from build123d import *

# Parameters (mm, degrees)
SKETCH1_R           = 11
SKETCH1_R_2         = 10
SKETCH1_R_3         = 1.75
SKETCH1_W           = 4
SKETCH1_H           = 20
BOSS_EXTRUDE1_DEPTH = 4


with BuildPart() as part:
    # Sketch1 → Boss-Extrude1 (new body)
    with BuildSketch(Plane(origin=(0, 0, 0), x_dir=(0, 0, -1), z_dir=(1, 0, 0))):
        Polygon((-20, 170.087118875), (20, 170.087118875), (75, 72.036415883), (75, -3.912881125), (55, -3.912881125), (55, 0.087118875), (10, 0.087118875), (10, -3.912881125), (-10, -3.912881125), (-10, 0.087118875), (-55, 0.087118875), (-55, -3.912881125), (-75, -3.912881125), (-75, 72.036415883), align=None)
        with Locations((0, 30.087118875)):
            Circle(SKETCH1_R, mode=Mode.SUBTRACT)
        with Locations((0, 140.087118875)):
            Circle(SKETCH1_R_2, mode=Mode.SUBTRACT)
        with Locations((-15.909902577, 45.997021452)):
            Circle(SKETCH1_R_3, mode=Mode.SUBTRACT)
        with Locations((-15.909902577, 14.177216298)):
            Circle(SKETCH1_R_3, mode=Mode.SUBTRACT)
        with Locations((15.909902577, 14.177216298)):
            Circle(SKETCH1_R_3, mode=Mode.SUBTRACT)
        with Locations((15.909902577, 45.997021452)):
            Circle(SKETCH1_R_3, mode=Mode.SUBTRACT)
        with BuildLine():
            Line((-10, 112.587118875), (10, 112.587118875))
            ThreePointArc((10, 112.587118875), (17.5, 105.087118875), (10, 97.587118875))
            Line((10, 97.587118875), (-10, 97.587118875))
            ThreePointArc((-10, 97.587118875), (-17.5, 105.087118875), (-10, 112.587118875))
        make_face(mode=Mode.SUBTRACT)
        with BuildLine():
            Line((-25, 82.587118875), (25, 82.587118875))
            ThreePointArc((25, 82.587118875), (32.5, 75.087118875), (25, 67.587118875))
            Line((25, 67.587118875), (-25, 67.587118875))
            ThreePointArc((-25, 67.587118875), (-32.5, 75.087118875), (-25, 82.587118875))
        make_face(mode=Mode.SUBTRACT)
        with Locations((-50, 15.087118875)):
            Rectangle(SKETCH1_W, SKETCH1_H, mode=Mode.SUBTRACT)
        with Locations((50, 15.087118875)):
            Rectangle(SKETCH1_W, SKETCH1_H, mode=Mode.SUBTRACT)
        with Locations((-50, 61.549860891)):
            Rectangle(SKETCH1_W, SKETCH1_H, mode=Mode.SUBTRACT)
        with Locations((50, 61.549860891)):
            Rectangle(SKETCH1_W, SKETCH1_H, mode=Mode.SUBTRACT)
    extrude(amount=BOSS_EXTRUDE1_DEPTH)


solid = part.part
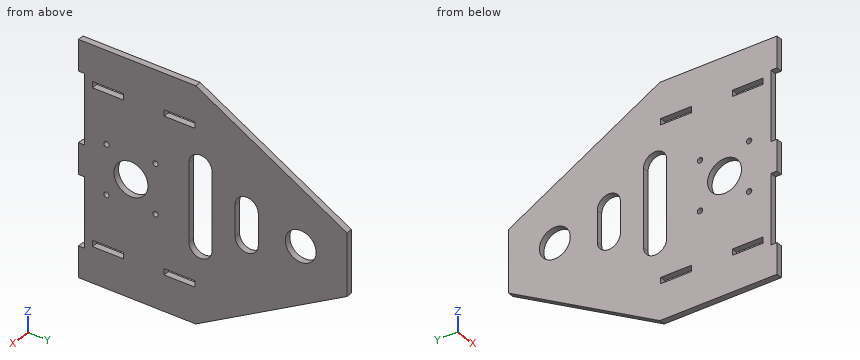
The model under review builds one solid part; all positions refer to its coordinate system, in mm. Round coordinates to 2 decimals unless told otherwise and drop trailing zeros. Write each loop counter-clockwise with the first axis right and the second up, starting at its lowest first coordinate (ties: lowest second). Pieces come first, ordered by that corner, then holes. Notation, with made-up numbers: (3, 24) - (19, 24) arc R20 cw to (19, 38) - close; hole circle Ø9 at (-27, 3.5). An arc over 180 degrees is marked (long way). One line per item, written item: value. Start each with the question number.
1. Consider section A-A on z = 0. Write out the cut boundary in (x, y).
2. Consider section D-D on x = 1.3. State how many separate pieces and enclosed holes the cut face has, and give its area (3 significant figures).
3. Clearance check with flat-ended pins moving along their axes: P1, Ø17.5, axis at y = 30.09, z = 0, coming from the +X side; P2, Ø2, axis at x = 2.5, z = -50, coming from the -Y side; P3, Ø1, axis at x = 3, z = 36, coming from the +Y side; P4, Ø2, axis at x = 1.5, z = -49.5, coming from the +Y side. State where each tip first meets the part, or that it passes through.
4. To check wall thickness, follow L1, parallel to Z at x = 2.1, y = 59; L2, parallel to Y at x = 1.3, z = 0; L3, parallel to Y at x = 1.8, z = -14.5. State the ranges of each line that lie inside material, in increasing order. Write a range as from..to.
5. Consider section C-C on y = 135. Write out the cut boundary in (x, z), and give its area (3 significant figures).
6. Consider section B-B on y = 75. Write out the cut boundary in (x, z).
Checks:
1. outline: (0, -3.91) - (4, -3.91) - (4, 19.09) - (0, 19.09) - close; (0, 41.09) - (4, 41.09) - (4, 67.59) - (0, 67.59) - close; (0, 82.59) - (4, 82.59) - (4, 97.59) - (0, 97.59) - close; (0, 112.59) - (4, 112.59) - (4, 130.09) - (0, 130.09) - close; (0, 150.09) - (4, 150.09) - (4, 170.09) - (0, 170.09) - close
2. separate pieces: 1
2. enclosed holes: 12
2. area: 17,900 mm^2
3. P1: passes through
3. P2: stops at y = 0.09
3. P3: stops at y = 142.45
3. P4: stops at y = 119.28
4. L1: z = -75..-52, -48..48, 52..75
4. L2: y = -3.91..19.09, 41.09..67.59, 82.59..97.59, 112.59..130.09, 150.09..170.09
4. L3: y = 0.09..13.14, 15.21..44.96, 47.03..67.59, 82.59..99.09, 111.09..170.09
5. outline: (0, -39.68) - (4, -39.68) - (4, -8.61) - (0, -8.61) - close; (0, 8.61) - (4, 8.61) - (4, 39.68) - (0, 39.68) - close
5. area: 249 mm^2
6. outline: (0, -73.34) - (4, -73.34) - (4, -32.5) - (0, -32.5) - close; (0, 32.5) - (4, 32.5) - (4, 73.34) - (0, 73.34) - close
